Source: three-view drawing plus pictorial views. Frame: mm from the lowest corner of the part. A direction names the side the tool comes from. Give positions to 0.01 mm unless a question says otherwise; leave off trailing zeros. Order: outer loops, then holes, each group sorted by start corner. A loop starts at its lowest first (then second) coordinate and runs counter-clockwise, first axis right, second up. Notation, with made-up numbers: (-19, 40.5) -> (26, 40.5) arc R3 ccw to (26, 44.5) -> close; hole circle Ø9 at (-30, 8). An arc over 180 degrees is marked (long way). Answer in a Markdown table with one row per item. Add a question column.
Q1. Cut plane A-A on x = 142.5. Return the cut outline in (y, z), and give its area (3 significant figures).
Q2. Line query: line 1 along Z through (x, y) = (142, 26); line 2 along Z through (x, y) = (142.5, 15). Output: solid intervals per line, ascending. Write a range as from..to.
Q3. Pull-direction query (Z, two-part tool) for the marked faces 3, 4, 5 and 6; classes: +Z half, -Z half, draft (parallel to the pull), parting line (faces both ways), or undercut.
Q4. Cut plane B-B on z = 142.5. Return the cut outline in (x, y), and give its area (3 significant figures).
Q5. Cut plane D-D on y = 16.5. Return the cut outline in (x, z), and give its area (3 significant figures).
Q6. Cut plane C-C on y = 58. Return the cut outline in (x, z), and give its area (3 significant figures).
Q7. Set-up query: the marked faces 1 and 2. Return all of +Z, -Z, +X, -X, +Y, -Y with unobstructed straight access to the full face (end or side cutting, diameter ignored); none if empty.
Q8. Contact query for flat-ended pins moving along their axis: P1, Ø12, axis at y = 10.5, z = 103, coming from the -X side; P2, Ø12, axis at y = 46.5, z = 52, coming from the -X side; P3, Ø3, axis at x = 63, y = 20.5, coming from the -Z side. Output: stop coordinate, or through.
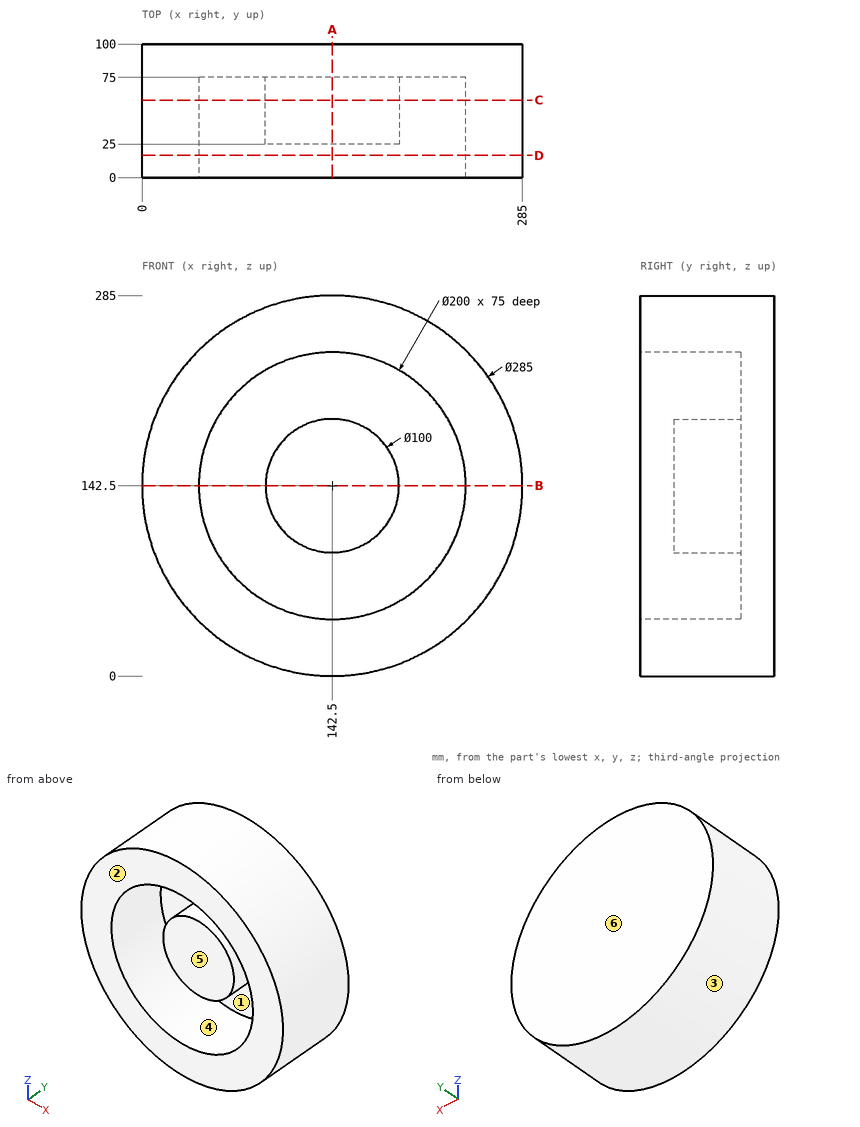
Completed:
| question | item | result |
|---|---|---|
| 1 | outline | (0, 0) -> (100, 0) -> (100, 285) -> (0, 285) -> (0, 242.5) -> (75, 242.5) -> (75, 192.5) -> (25, 192.5) -> (25, 92.5) -> (75, 92.5) -> (75, 42.5) -> (0, 42.5) -> close |
| 1 | area | 18,500 mm² |
| 2 | line 1 | z = 0..42.5, 92.5..192.5, 242.5..285 |
| 2 | line 2 | z = 0..42.5, 242.5..285 |
| 3 | face 3 | parting line |
| 3 | face 4 | undercut |
| 3 | face 5 | undercut |
| 3 | face 6 | draft |
| 4 | outline | (0, 0) -> (42.5, 0) -> (42.5, 75) -> (92.5, 75) -> (92.5, 25) -> (192.5, 25) -> (192.5, 75) -> (242.5, 75) -> (242.5, 0) -> (285, 0) -> (285, 100) -> (0, 100) -> close |
| 4 | area | 18,500 mm² |
| 5 | outline | circle Ø285 at (142.5, 142.5); hole circle Ø200 at (142.5, 142.5) |
| 5 | area | 32,400 mm² |
| 6 | outline | circle Ø285 at (142.5, 142.5); circle Ø100 at (142.5, 142.5); hole circle Ø200 at (142.5, 142.5) |
| 6 | area | 40,200 mm² |
| 7 | face 1 | -Y |
| 7 | face 2 | +Z, -Z, +X, -X, -Y |
| 8 | P1 | stops at x = 3.99 |
| 8 | P2 | stops at x = 27.76 |
| 8 | P3 | stops at z = 23.24 |
